Could you check a few things on this model? Use its own coordinates, in mm. A direction names the side the tool comes from. Give positions to 0.01 mm unless a question says otherwise; leave off trailing zeros. Order: outer loops, then holes, each group sorted by start corner. A loop starts at its lowest first (then second) coordinate and runs counter-clockwise, first axis right, second up. Notation, with made-up numbers: (6, -4) - (46, -4) arc R29 ccw to (46, 27) - close; hole circle Ø8 at (39.5, -38.5). An arc over 180 degrees is marked (long way). One line per question, with ' | ' between items. Start each with the question number.
1. Imagine slicing it at A-A (x = -8.5). Please give me the cut outline in (y, z).
2. Imagine slicing it at D-D (x = -28). Give the number of separate pieces and of enclosed holes in the cut face, and give its area (3 significant figures).
3. If we mould it in two halves opening along X, with no side actions, what happens to faces 1 (the flat face through (-8, 1, 0)), 2 (the flat face through (-16, 4, -13)), 3 (the flat face through (-33, 3, -14)), 4 (the flat face through (0, 2, -16))? For each: released by +X, released by -X, zero draft, split by the parting line, or undercut.
4. Which directions (+Z, -Z, +X, -X, +Y, -Y) give clear straight access to the entire face, cutting with the end or side of a thin tool? Please do faces 5 (the flat face through (-9, 4, -32)), 6 (the cylindrical face through (-8.825, 1.232, -6.036)), 7 (the cylindrical face through (-22.62, 8.2, -18.92)).
5. Imagine slicing it at C-C (y = 3.5). Please give me the cut outline in (x, z), and give its area (3 significant figures).
6. I need wall thicknesses on probe 1 along Z at (x, y) = (-27.5, 4); probe 2 along X at (y, z) = (7.5, -20); probe 3 along X at (y, z) = (3.75, -15). Which ranges of each line are inside material? Lowest first, please. Write a range as from..to.
7. Imagine slicing it at B-B (z = -26.5). Please give me the cut outline in (x, y).
8. For P1, Ø5.5, axis at x = -7.5, y = 3.5, coming from the +Z side; P2, Ø2, axis at x = -5, y = 4.5, coming from the +Z side; P3, Ø1, axis at x = -14, z = -21, coming from the +Y side, each with a flat end and sliding along its axis, tell me the tip position at first contact or that it passes through.
```python
from build123d import *

# Parameters (mm, degrees)
SKETCH1_W                = 33
SKETCH1_H                = 33
BOSS_EXTRUDE1_DEPTH      = 5
SKETCH2_W                = 15
SKETCH2_H                = 32
CUT_EXTRUDE1_DEPTH       = 2.5
SKETCH4_W                = 17
SKETCH4_H                = 5
BOSS_EXTRUDE3_DEPTH      = 5
SKETCH3_R                = 5
SKETCH3_R_2              = 2.5
BOSS_EXTRUDE4_DEPTH      = 6.5
CUT_EXTRUDE4_START       = -5
CUT_EXTRUDE4_OUTLINE_R   = 2.5
CUT_EXTRUDE4_OUTLINE_R_2 = 1.5
CUT_EXTRUDE4_DEPTH       = 5


# Read off the part's stored shape, not the designer's step: Cut-Extrude4
with BuildPart() as part:
    # Sketch1 → Boss-Extrude1 (new body)
    with BuildSketch(Plane(origin=(0, 0, 0), x_dir=(1, 0, 0), z_dir=(0, 1, 0))):
        with Locations((-16.5, 16.5)):
            Rectangle(SKETCH1_W, SKETCH1_H)
    extrude(amount=BOSS_EXTRUDE1_DEPTH)

    # Sketch2 → Cut-Extrude1 (cut)
    with BuildSketch(Plane(origin=(0, 5, 0), x_dir=(1, 0, 0), z_dir=(0, 1, 0))):
        with Locations((-8.5, 16)):
            Rectangle(SKETCH2_W, SKETCH2_H)
    extrude(amount=-CUT_EXTRUDE1_DEPTH, mode=Mode.SUBTRACT)

    # Sketch4 → Boss-Extrude3 (add)
    with BuildSketch(Plane(origin=(0, 5, 0), x_dir=(1, 0, 0), z_dir=(0, 1, 0))):
        with Locations((-24.5, -2.5)):
            Rectangle(SKETCH4_W, SKETCH4_H)
    extrude(amount=-BOSS_EXTRUDE3_DEPTH)

    # Sketch3 → Boss-Extrude4 (add)
    # profile 1 of 2: a face of its own
    with BuildSketch(Plane(origin=(0, 5, 0), x_dir=(1, 0, 0), z_dir=(0, 1, 0))):
        with Locations(Location((-27.5, 20, 0), (0, 0, 90))):
            Circle(SKETCH3_R)
        with Locations(Location((-27.5, 20, 0), (0, 0, 90))):
            Circle(SKETCH3_R_2, mode=Mode.SUBTRACT)
    # profile 2 of 2: a face of its own
    with BuildSketch(Plane(origin=(0, 5, 0), x_dir=(1, 0, 0), z_dir=(0, 1, 0))):
        with Locations(Location((-27.5, 0, 0), (0, 0, 270))):
            Circle(SKETCH3_R)
        with Locations(Location((-27.5, 0, 0), (0, 0, 90))):
            Circle(SKETCH3_R_2, mode=Mode.SUBTRACT)
    extrude(amount=BOSS_EXTRUDE4_DEPTH)

    # Cut-Extrude4 outline → Cut-Extrude4 (cut)
    with BuildSketch(Plane(origin=(0, 5, 0), x_dir=(1, 0, 0), z_dir=(0, 1, 0)).offset(CUT_EXTRUDE4_START)):
        with Locations((-27.5, 20)):
            Circle(CUT_EXTRUDE4_OUTLINE_R)
        with Locations((-27.5, 0)):
            Circle(CUT_EXTRUDE4_OUTLINE_R)
        with Locations((-8.5, 7.5)):
            Circle(CUT_EXTRUDE4_OUTLINE_R_2)
    extrude(amount=CUT_EXTRUDE4_DEPTH, mode=Mode.SUBTRACT)


solid = part.part
```
Results found:
1) outline: (0, -33) - (5, -33) - (5, -32) - (2.5, -32) - (2.5, -9) - (0, -9) - close; (0, -6) - (2.5, -6) - (2.5, 0) - (0, 0) - close
2) separate pieces: 3 | enclosed holes: 0 | area: 207 mm2
3) face 1: zero draft | face 2: undercut | face 3: released by -X | face 4: released by +X
4) face 5: +Z, +Y | face 6: +Y, -Y | face 7: +Y
5) outline: (-33, -33) - (0, -33) - (0, 0) - (-1, 0) - (-1, -32) - (-16, -32) - (-16, 5) - (-33, 5) - close; hole circle Ø5 at (-27.5, -20); hole circle Ø5 at (-27.5, 0) | area: 655 mm2
6) probe 1: z = -33..-22.5, -17.5..-2.5, 2.5..5 | probe 2: x = -32.5..-30, -25..-22.5 | probe 3: x = -33..-16, -1..0
7) outline: (-33, 0) - (0, 0) - (0, 5) - (-1, 5) - (-1, 2.5) - (-16, 2.5) - (-16, 5) - (-33, 5) - close
8) P1: stops at z = 0 | P2: stops at z = -32 | P3: stops at y = 2.5
